```python
from build123d import *

# Parameters (mm, degrees)
F0_W     = 5
F0_H     = 3
F1_DEPTH = 5
F2_DEPTH = 23


with BuildPart() as f1:
    # F0 (on Top) → F1 (new body)
    with BuildSketch(Plane.XY):
        Rectangle(F0_W, F0_H)
        with BuildLine():
            Line((-1, 0.5), (1, 0.5))
            ThreePointArc((1, 0.5), (1.353553, 0.353553), (1.5, 0))
            ThreePointArc((1.5, 0), (1.353553, -0.353553), (1, -0.5))
            Line((1, -0.5), (-1, -0.5))
            ThreePointArc((-1, -0.5), (-1.5, 0), (-1, 0.5))
        make_face(mode=Mode.SUBTRACT)
        with BuildLine():
            ThreePointArc((1, -0.5), (0.646447, -0.353553), (0.5, 0))
            ThreePointArc((0.5, 0), (0.646447, 0.353553), (1, 0.5))
            Line((1, 0.5), (-1, 0.5))
            ThreePointArc((-1, 0.5), (-0.646447, 0.353553), (-0.5, 0))
            ThreePointArc((-0.5, 0), (-0.646447, -0.353553), (-1, -0.5))
            Line((-1, -0.5), (1, -0.5))
        make_face()
    extrude(amount=F1_DEPTH)

    # F0 (on Top) → F2 (join)
    with BuildSketch(Plane.XY):
        with BuildLine():
            ThreePointArc((1, -0.5), (0.646447, -0.353553), (0.5, 0))
            ThreePointArc((0.5, 0), (0.646447, 0.353553), (1, 0.5))
            Line((1, 0.5), (-1, 0.5))
            ThreePointArc((-1, 0.5), (-0.646447, 0.353553), (-0.5, 0))
            ThreePointArc((-0.5, 0), (-0.646447, -0.353553), (-1, -0.5))
            Line((-1, -0.5), (1, -0.5))
        make_face()
    extrude(amount=F2_DEPTH)


solid = f1.part
```
Work out the finished part from the listing and answer in its coordinate system (mm). A direction names the side the tool comes from. Give positions to 0.01 mm unless a question says otherwise; leave off trailing zeros. Order: outer loops, then holes, each group sorted by start corner. A loop starts at its lowest first (then second) coordinate and runs counter-clockwise, first axis right, second up. Notation, with made-up numbers: M 50,-39.75 L 70,-39.75 A25 cw 70,-23.75 Z; hole C 89,10.25 d1. An arc over 180 degrees is marked long. Return JSON: item names as keys, results as strings.
1) Each of these flat-tipped pins is pushed along its axis until it touches: pin 1 (1.6 mm diameter, centred on x = 0, z = 18.5, fed in from +Y); pin 2 (1 mm diameter, centred on x = 0.5, z = 9.5, fed in from -Y). Where does it stop, or does it pass through?
Resolved:
{"pin 1": "y = 0.5", "pin 2": "y = -0.5"}
2) A tool of negligible diameter and unlimited length cuts with its end or side. For faces 1 (the flat face through (0, 0.5, 14)), 2 (the flat face through (0, -1.5, 2)), 3 (the flat face through (0, -0.5, 14)), from which of +Z, -Z, +X, -X, +Y, -Y can it reach the whole face along a straight path? Write none if from no direction.
Resolved:
{"face 1": "+Z, +X, -X, +Y", "face 2": "+Z, -Z, +X, -X, -Y", "face 3": "+Z, +X, -X, -Y"}
3) Straight lines are drawn through the part: line 1 along Y through (x, z) = (-0.15, 6); line 2 along Z through (x, y) = (1.15, -0.6); line 3 along Y through (x, z) = (1.35, 1.75). For each, find the intervals that lie inside material, in ascending order. Write a range as [from, to].
Resolved:
{"line 1": "[-0.5, 0.5]", "line 2": "[0, 5]", "line 3": "[-1.5, -0.36], [0.36, 1.5]"}
4) Section B-B, the plane z = 21.25 is taken. Write down the section's boundary in (x, y), plus the area to 3 significant figures.
Resolved:
{"outline": "M -1,-0.5 L 1,-0.5 A0.5 cw 0.5,0 A0.5 cw 1,0.5 L -1,0.5 A0.5 cw -0.5,0 A0.5 cw Z", "area": "1.21 mm^2"}
5) Section C-C, the plane y = -1.05 is taken. Write down the section's boundary in (x, z), plus the area to 3 significant figures.
Resolved:
{"outline": "M -2.5,0 L 2.5,0 L 2.5,5 L -2.5,5 Z", "area": "25.0 mm^2"}
6) Section D-D, the plane x = -1.9 is taken. Write down the section's boundary in (y, z), plus the area to 3 significant figures.
Resolved:
{"outline": "M -1.5,0 L 1.5,0 L 1.5,5 L -1.5,5 Z", "area": "15.0 mm^2"}
7) Section A-A, the plane x = 0.7 is taken. Write down the section's boundary in (y, z).
Resolved:
{"outline": "M -1.5,0 L -0.4,0 L -0.4,23 L -0.5,23 L -0.5,5 L -1.5,5 Z; M 0.4,0 L 1.5,0 L 1.5,5 L 0.5,5 L 0.5,23 L 0.4,23 Z"}
